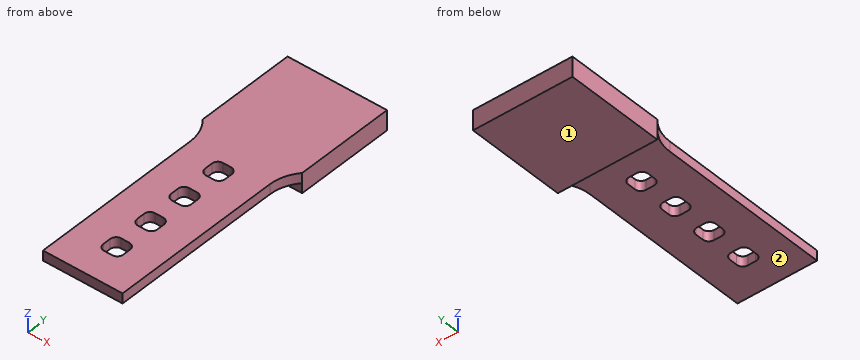
Autodesk Inventor part; units mm, degrees
ref_plane "YZ Plane" through (0, 0, 0) normal (1, 0, 0) x (0, 1, 0)
ref_plane "XZ Plane" through (0, 0, 0) normal (0, 1, 0) x (-1, 0, 0)
ref_plane "XY Plane" through (0, 0, 0) normal (0, 0, 1) x (1, 0, 0)
sketch "Boceto1" plane through (0, 0, 0) normal (0, 0, 1) x (1, 0, 0)
  line L0 (-20, -50) -> (20, -50)
  line L1 (20, -50) -> (20, 50)
  line L2 (20, 50) -> (-20, 50)
  line L3 (-20, 50) -> (-20, -50)
  line L4 (-20, -50) -> (20, 50) construction
  line L5 (20, -50) -> (-20, 50) construction
  line L6 (-25, 100) -> (25, 100)
  line L7 (25, 100) -> (25, 50)
  line L8 (25, 50) -> (-25, 50)
  line L9 (-25, 50) -> (-25, 100)
  line L10 (-25, 100) -> (25, 50) construction
  line L11 (25, 100) -> (-25, 50) construction
  line L12 (-25, -50) -> (25, -50)
  line L13 (25, -50) -> (25, -100)
  line L14 (25, -100) -> (-25, -100)
  line L15 (-25, -100) -> (-25, -50)
  line L16 (-25, -50) -> (25, -100) construction
  line L17 (25, -50) -> (-25, -100) construction
  line L18 (0, 50) -> (0, 30) construction
  line L19 (0, 30) -> (0, 10) construction
  line L20 (0, 10) -> (0, -10) construction
  line L21 (0, -10) -> (0, -30) construction
  line L22 (0, -30) -> (0, -50) construction
  line L23 (0, 30) -> (0, 30) construction
  line L24 (0, 10) -> (0, 10) construction
  line L25 (0, -10) -> (0, -10) construction
  line L26 (0, -30) -> (0, -30) construction
  line L27 (2, 35) -> (-2, 35)
  line L28 (-5, 32) -> (-5, 28)
  line L29 (-2, 25) -> (2, 25)
  line L30 (5, 28) -> (5, 32)
  line L31 (5, 35) -> (-5, 25) construction
  line L32 (-5, 35) -> (5, 25) construction
  line L33 (2, 15) -> (-2, 15)
  line L34 (-5, 12) -> (-5, 8)
  line L35 (-2, 5) -> (2, 5)
  line L36 (5, 8) -> (5, 12)
  line L37 (5, 15) -> (-5, 5) construction
  line L38 (-5, 15) -> (5, 5) construction
  line L39 (2, -5) -> (-2, -5)
  line L40 (-5, -8) -> (-5, -12)
  line L41 (-2, -15) -> (2, -15)
  line L42 (5, -12) -> (5, -8)
  line L43 (5, -5) -> (-5, -15) construction
  line L44 (-5, -5) -> (5, -15) construction
  line L45 (2, -25) -> (-2, -25)
  line L46 (-5, -28) -> (-5, -32)
  line L47 (-2, -35) -> (2, -35)
  line L48 (5, -32) -> (5, -28)
  line L49 (5, -25) -> (-5, -35) construction
  line L50 (-5, -25) -> (5, -35) construction
  line L51 (0, 30) -> (0, 10) construction
  arc A0 (-2, 35) -> (-5, 32) centre (-2, 32) ccw
  arc A1 (5, 32) -> (2, 35) centre (2, 32) ccw
  arc A2 (2, 25) -> (5, 28) centre (2, 28) ccw
  arc A3 (-5, 28) -> (-2, 25) centre (-2, 28) ccw
  arc A4 (-2, 15) -> (-5, 12) centre (-2, 12) ccw
  arc A5 (-5, 8) -> (-2, 5) centre (-2, 8) ccw
  arc A6 (2, 5) -> (5, 8) centre (2, 8) ccw
  arc A7 (5, 12) -> (2, 15) centre (2, 12) ccw
  arc A8 (5, -8) -> (2, -5) centre (2, -8) ccw
  arc A9 (-2, -5) -> (-5, -8) centre (-2, -8) ccw
  arc A10 (-5, -12) -> (-2, -15) centre (-2, -12) ccw
  arc A11 (2, -15) -> (5, -12) centre (2, -12) ccw
  arc A12 (5, -28) -> (2, -25) centre (2, -28) ccw
  arc A13 (2, -35) -> (5, -32) centre (2, -32) ccw
  arc A14 (-5, -32) -> (-2, -35) centre (-2, -32) ccw
  arc A15 (-2, -25) -> (-5, -28) centre (-2, -28) ccw
  point P0 (0, 0)
  point P1 (0, 75)
  point P2 (0, -75)
  dimension "d0" = 40
  dimension "d1" = 100
  dimension "d2" = 50
  dimension "d3" = 50
  dimension "d4" = 50
  dimension "d5" = 50
  dimension "d6" = 20
  dimension "d7" = 20
  dimension "d8" = 20
  dimension "d9" = 20
  dimension "d10" = 0
  dimension "d11" = 0
  dimension "d12" = 0
  dimension "d13" = 0
  dimension "d25" = 10
  dimension "d26" = 10
  dimension "d27" = 10
  dimension "d28" = 10
  dimension "d29" = 10
  dimension "d30" = 10
  dimension "d31" = 10
  dimension "d32" = 10
  dimension "d33" = 20
  dimension "d34" = 3
extrude "Extrusión1" add sketch "Boceto1" along normal blind 10 contours L3 L2 L1 L0 | L8 L9 L6 L7 L2
extrude "Extrusión2" cut sketch "Boceto1" along normal blind 5 contours L3 L2 L1 L0 | A1 L30 A2 L29 A3 L28 A0 L27 | A7 L36 A6 L35 A5 L34 A4 L33 | A8 L42 A11 L41 A10 L40 A9 L39 | A12 L48 A13 L47 A14 L46 A15 L45
fillet "Empalme3" radius 20 2 edges at (20, 50, 7.5) (-20, 50, 7.5)
properties material "MDF Tablero de fibras de densidad media"
Verification items for the finished model (mm, model axes). Face numbers are marked on the shaded views. A direction names the side the tool comes from. Coordinates: 2 decimals unless noted, no trailing zeros. Order: outer loops, then holes, each group sorted by start corner. A loop starts at its lowest first (then second) coordinate and runs counter-clockwise, first axis right, second up.
1. Scan lines: line 1 (Y direction, x = 1, z = 8.75); line 2 (X direction, y = 32, z = 8.75); line 3 (Y direction, x = -12.5, z = 4). Record each from-to range of solid material in increasing order.
Results found:
line 1: y = -50 to -35, -25 to -15, -5 to 5, 15 to 25, 35 to 100
line 2: x = -20 to -5, 5 to 20
line 3: y = 50 to 100
2. Sectioned sample at A-A, the plane x = 0.5. Record the cut outline in (y, z).
Results found:
outline: (-50, 5) - (-35, 5) - (-35, 10) - (-50, 10) - close; (-25, 5) - (-15, 5) - (-15, 10) - (-25, 10) - close; (-5, 5) - (5, 5) - (5, 10) - (-5, 10) - close; (15, 5) - (25, 5) - (25, 10) - (15, 10) - close; (35, 5) - (50, 5) - (50, 0) - (100, 0) - (100, 10) - (35, 10) - close
3. Go/stop test with flat-tipped pins: pin 1 Ø1.5 at (y, z) = (-15, 6.5) entering from +X; pin 2 Ø5.5 at (y, z) = (7, 7) entering from -X; pin 3 Ø2.5 at (x, z) = (12, 2) entering from -Y. Record where each tip stops, or that it passes through.
Results found:
pin 1: stops at x = 20
pin 2: stops at x = -20
pin 3: stops at y = 50
4. Sectioned sample at C-C, the plane y = -21. Record the cut outline in (x, z).
Results found:
outline: (-20, 5) - (20, 5) - (20, 10) - (-20, 10) - close
5. Sectioned sample at D-D, the plane z = 3. Record the cut outline in (x, y), and give its area (3 significant figures).
Results found:
outline: (-25, 50) - (25, 50) - (25, 100) - (-25, 100) - close
area: 2,500 mm2
6. Sectioned sample at B-B, the plane x = 7.5. Record the cut outline in (y, z), and give its area (3 significant figures).
Results found:
outline: (-50, 5) - (50, 5) - (50, 0) - (100, 0) - (100, 10) - (-50, 10) - close
area: 1,000 mm2
7. Set-up check for the marked faces 1 and 2: record each of +Z, -Z, +X, -X, +Y, -Y from which the full face is reachable in a straight line by a thin tool's end or side.
Results found:
face 1: -Z, +X, -X, +Y, -Y
face 2: -Z, +X, -X, -Y
